Autodesk Inventor part; units mm, degrees
ref_plane "Plan de construction1" through (-33.0415, -128.424, -137.979) normal (0, -1, 0) x (1, 0, 0)
ref_plane "YZ Plane" through (0, 0, 0) normal (1, 0, 0) x (0, 1, 0)
ref_plane "XZ Plane" through (0, 0, 0) normal (0, 1, 0) x (-1, 0, 0)
sketch "Esquisse1" plane through (0, 0, 0) normal (0, 0, 1) x (1, 0, 0)
  circle A0 centre (-5.13, -4.2) radius 1.738
  circle A1 centre (43.13, -2.93) radius 1.738
  circle A2 centre (10.11, -55) radius 1.738
  circle A3 centre (51.1638, -91.424) radius 1.5682
  circle A4 centre (-13.5548, -91.424) radius 1.5682
  line L0 (-5.13, -4.2) -> (43.13, -2.93) construction
  line L1 (-5.0248, -8.1986) -> (43.2352, -6.9286)
  line L2 (43.0248, 1.0686) -> (-5.2352, -0.2014)
  arc A5 (-5.2352, -0.2014) -> (-5.0248, -8.1986) centre (-5.13, -4.2) ccw
  arc A6 (43.2352, -6.9286) -> (43.0248, 1.0686) centre (43.13, -2.93) ccw
  arc A7 (-1.2987, -3.0506) -> (-8.9613, -5.3494) centre (-5.13, -4.2) ccw
  arc A8 (46.508, -5.0722) -> (39.752, -0.7878) centre (43.13, -2.93) ccw
  arc A9 (-16.909, -89.2447) -> (-10.2005, -93.6032) centre (-13.5548, -91.424) ccw
  arc A10 (48.5091, -94.4161) -> (53.8185, -88.4319) centre (51.1638, -91.424) ccw
  line L3 (43.13, -2.93) -> (51.1638, -91.424) construction
  line L4 (39.1464, -3.2916) -> (47.1802, -91.7856)
  line L5 (55.1474, -91.0623) -> (47.1136, -2.5684)
  arc A11 (47.1136, -2.5684) -> (39.1464, -3.2916) centre (43.13, -2.93) ccw
  arc A12 (47.1802, -91.7856) -> (55.1474, -91.0623) centre (51.1638, -91.424) ccw
  line L6 (-5.13, -4.2) -> (-13.5548, -91.424) construction
  line L7 (-1.1485, -4.5846) -> (-9.5733, -91.8085)
  line L8 (-17.5362, -91.0394) -> (-9.1115, -3.8154)
  arc A13 (-1.1485, -4.5846) -> (-9.1115, -3.8154) centre (-5.13, -4.2) ccw
  arc A14 (-17.5362, -91.0394) -> (-9.5733, -91.8085) centre (-13.5548, -91.424) ccw
  line L9 (-13.5548, -91.424) -> (51.1638, -91.424) construction
  line L10 (-13.5548, -95.424) -> (51.1638, -95.424)
  line L11 (51.1638, -87.424) -> (-13.5548, -87.424)
  arc A15 (-13.5548, -87.424) -> (-13.5548, -95.424) centre (-13.5548, -91.424) ccw
  arc A16 (51.1638, -95.424) -> (51.1638, -87.424) centre (51.1638, -91.424) ccw
  point P0 (0, 0)
  point P1 (19, -3.565)
  point P2 (2.49, -29.6)
  point P3 (-1.7224, -73.212)
  point P4 (30.6369, -73.212)
  point P5 (47.1469, -47.177)
  point P6 (-9.3424, -47.812)
  point P7 (18.8045, -91.424)
  point P8 (39.4855, -7.0273)
  point P9 (46.7842, -87.424)
  point P10 (-9.1498, -87.424)
  point P11 (-1.4886, -8.1056)
  point P12 (-9.1115, -3.8154)
  point P13 (51.1638, -95.424)
  point P14 (47.1136, -2.5684)
  dimension "d2" = 8
  dimension "d3" = 8
  dimension "d5" = 8
  dimension "d6" = 8
extrude "Extrusion1" add sketch "Esquisse1" along normal blind 4 contours A5 A7 A13 L7 L1 | L1 L7 L11 A15 A9 L8 A5 | L7 A13 A7 L2 A8 A11 L4 L1 | L4 A11 A8 A6 L1 | L1 A6 L5 A10 A16 L11 L4 | L11 L4 A12 A10 L10 A9 A14 L7 | L7 A14 A9 A15 L11 | L11 A16 A10 A12 L4
fillet "Congé1" radius 19 2 edges at (-1.4886, -8.1056, 2) (39.4855, -7.0273, 2)
sketch "Esquisse2" plane through (0, 0, 0) normal (0, 0, -1) x (-1, 0, 0)
  arc A0 (9.1115, -3.8154) -> (5.2352, -0.2014) centre (5.13, -4.2) ccw
  line L0 (-43.0248, 1.0686) -> (5.2352, -0.2014)
  arc A1 (-43.0248, 1.0686) -> (-47.1136, -2.5684) centre (-43.13, -2.93) ccw
  line L1 (-55.1474, -91.0623) -> (-47.1136, -2.5684)
  arc A2 (-55.1474, -91.0623) -> (-51.1638, -95.424) centre (-51.1638, -91.424) ccw
  line L2 (13.5548, -95.424) -> (-51.1638, -95.424)
  arc A3 (13.5548, -95.424) -> (17.5362, -91.0394) centre (13.5548, -91.424) ccw
  line L3 (9.1115, -3.8154) -> (17.5362, -91.0394)
  arc A4 (-21.6744, -7.496) -> (-41.0964, -24.7716) centre (-22.1742, -26.4894) ccw
  line L4 (-15.3081, -7.6635) -> (-21.6744, -7.496)
  arc A5 (3.104, -24.8303) -> (-15.3081, -7.6635) centre (-15.808, -26.657) ccw
  line L5 (9.1498, -87.424) -> (3.104, -24.8303)
  line L6 (-46.7842, -87.424) -> (9.1498, -87.424)
  line L7 (-41.0964, -24.7716) -> (-46.7842, -87.424)
  circle A6 centre (5.13, -4.2) radius 1.738
  circle A7 centre (13.5548, -91.424) radius 1.5682
  circle A8 centre (-43.13, -2.93) radius 1.738
  circle A9 centre (-51.1638, -91.424) radius 1.5682
  line L8 (-41.0964, -24.7716) -> (-46.7842, -87.424)
  line L9 (-46.7842, -87.424) -> (-47.5105, -95.424)
  line L10 (-55.1474, -91.0623) -> (-47.1136, -2.5684)
  line L11 (-46.7842, -87.424) -> (9.1498, -87.424)
  line L12 (-46.7842, -87.424) -> (-54.8171, -87.424)
  line L13 (9.1498, -87.424) -> (9.9225, -95.424)
  line L14 (9.1498, -87.424) -> (17.187, -87.424)
  point P0 (0, 0)
extrude "Extrusion2" add sketch "Esquisse2" along normal blind 20 contours L3 A3 L2 L13 L14 | L9 L2 A2 L1 L12
sketch "Esquisse3" plane through (-13.5548, -95.424, 4) normal (0, -1, 0) x (1, 0, 0)
  line L0 (3.6323, -4) -> (61.0652, -4)
  line L1 (61.0652, -4) -> (61.0652, -24)
  line L2 (64.7185, -24) -> (61.0652, -24)
  line L3 (64.7185, -24) -> (64.7185, 0)
  line L4 (0, 0) -> (64.7185, 0)
  line L5 (0, -24) -> (0, 0)
  line L6 (3.6323, -24) -> (0, -24)
  line L7 (3.6323, -4) -> (3.6323, -24)
  line L8 (0, -24) -> (0, 0)
  line L9 (-3.9815, 0) -> (0, 0)
  line L10 (-3.9815, -24) -> (-3.9815, 0)
  line L11 (0, -24) -> (-3.9815, -24)
  line L12 (68.7022, -24) -> (68.7022, 0)
  line L13 (64.7185, 0) -> (68.7022, 0)
  line L14 (64.7185, -24) -> (64.7185, 0)
  line L15 (68.7022, -24) -> (64.7185, -24)
  point P0 (13.5548, -4)
  point P1 (0, 0)
  point P2 (64.7185, 0)
extrude "Extrusion3" add sketch "Esquisse3" along normal blind 25
sketch "Esquisse4" plane through (0, 0, 4) normal (0, 0, 1) x (1, 0, 0)
  arc A0 (-5.2352, -0.2014) -> (-9.1115, -3.8154) centre (-5.13, -4.2) ccw
  line L0 (-9.1115, -3.8154) -> (-17.5362, -91.0394)
  arc A1 (-17.5362, -91.0394) -> (-13.5548, -95.424) centre (-13.5548, -91.424) ccw
  line L1 (-13.5548, -95.424) -> (-17.5362, -95.424)
  line L2 (-17.5362, -95.424) -> (-17.5362, -120.424)
  line L3 (55.1474, -120.424) -> (-17.5362, -120.424)
  line L4 (55.1474, -95.424) -> (55.1474, -120.424)
  line L5 (55.1474, -95.424) -> (51.1638, -95.424)
  arc A2 (51.1638, -95.424) -> (55.1474, -91.0623) centre (51.1638, -91.424) ccw
  line L6 (55.1474, -91.0623) -> (47.1136, -2.5684)
  arc A3 (47.1136, -2.5684) -> (43.0248, 1.0686) centre (43.13, -2.93) ccw
  line L7 (43.0248, 1.0686) -> (-5.2352, -0.2014)
  line L8 (41.0964, -24.7716) -> (46.7842, -87.424)
  line L9 (46.7842, -87.424) -> (-9.1498, -87.424)
  line L10 (-9.1498, -87.424) -> (-3.104, -24.8303)
  arc A4 (15.3081, -7.6635) -> (-3.104, -24.8303) centre (15.808, -26.657) ccw
  line L11 (15.3081, -7.6635) -> (21.6744, -7.496)
  arc A5 (41.0964, -24.7716) -> (21.6744, -7.496) centre (22.1742, -26.4894) ccw
  circle A6 centre (-5.13, -4.2) radius 1.738
  circle A7 centre (-13.5548, -91.424) radius 1.5682
  circle A8 centre (43.13, -2.93) radius 1.738
  circle A9 centre (51.1638, -91.424) radius 1.5682
  line L12 (-17.5362, -91.0394) -> (-17.187, -87.424)
  line L13 (-17.5362, -95.424) -> (-17.5362, -91.0394)
  line L14 (55.1474, -91.0623) -> (55.1474, -95.424)
  point P0 (0, 0)
  point P1 (55.1474, -91.7856)
  point P2 (-17.5362, -91.8085)
extrude "Extrusion4" add sketch "Esquisse4" against normal up to surface (24 mm away) contours A1 L1 L13 | L14 L5 A2
sketch "Esquisse5" plane through (-13.5548, -120.424, 4) normal (0, -1, 0) x (1, 0, 0)
  line L0 (68.7022, 0) -> (-3.9815, 0)
  line L1 (-3.9815, 0) -> (-3.9815, -24)
  line L2 (68.7022, 0) -> (-3.9815, 0)
  line L3 (-3.9815, 0) -> (-3.9815, -24)
  line L4 (-3.9815, -24) -> (68.7022, -24)
  line L5 (68.7022, -24) -> (68.7022, 0)
  point P0 (13.5548, -4)
extrude "Extrusion5" add sketch "Esquisse5" along normal blind 3
sketch "Esquisse6" plane through (-13.5548, -120.424, 4) normal (0, 1, 0) x (1, 0, 0)
  circle A0 centre (52.3133, 6.979) radius 1.6
  circle A1 centre (52.3133, 16.979) radius 1.6
  circle A2 centre (42.3133, 16.979) radius 1.6
  circle A3 centre (42.3133, 6.979) radius 1.6
  circle A4 centre (32.3133, 6.979) radius 1.6
  circle A5 centre (32.3133, 16.979) radius 1.6
  circle A6 centre (22.3133, 16.979) radius 1.6
  circle A7 centre (22.3133, 6.979) radius 1.6
  circle A8 centre (12.3133, 6.979) radius 1.6
  circle A9 centre (12.3133, 16.979) radius 1.6
  point P0 (13.5548, 4)
ref_plane "Plan de construction1" through (-33.0415, -128.424, -137.979) normal (0, -1, 0) x (1, 0, 0)
extrude "Extrusion6" cut sketch "Esquisse6" against normal up to surface (8 mm away)
properties part number "holder"
Verification items for the finished model (mm, model axes). A direction names the side the tool comes from. Give positions to 0.01 mm unless a question says otherwise; leave off trailing zeros. Write each loop counter-clockwise with the first axis right and the second up, starting at its lowest first coordinate (ties: lowest second). Pieces come first, ordered by that corner, then holes. Notation, with made-up numbers: M 31.25,79.5 L 79.25,79.5 A22 cw 79.25,86.5 Z; hole C 87,-23.5 d10. An arc over 180 degrees is marked long. Write item = value, one per line.
(1) Sectioned sample at A-A (y = -115). Record the cut outline in (x, z).
Found:
outline = M -17.54,-20 L -9.92,-20 L -9.92,0 L 47.51,0 L 47.51,-20 L 55.15,-20 L 55.15,4 L -17.54,4 Z
(2) Go/stop test with flat-tipped pins: pin 1 Ø6 at (y, z) = (-113.5, -7.5) entering from +X; pin 2 Ø4 at (x, z) = (38.76, -2.98) entering from -Y; pin 3 Ø4 at (x, z) = (-12, -15) entering from +Y; pin 4 Ø4.5 at (x, y) = (-5.13, -4.2) entering from -Z. Record where each tip stops, or that it passes through.
Found:
pin_1 = 55.15
pin_2 = -123.42
pin_3 = -87.42
pin_4 = 0
(3) Sectioned sample at D-D (y = -85). Record the cut outline in (x, z).
Found:
outline = M -16.95,0 L -8.92,0 L -8.92,4 L -16.95,4 Z; M 46.56,0 L 54.6,0 L 54.6,4 L 46.56,4 Z
(4) Access from +Z, -Z, +X, -X, +Y, -Y to the whole of each face (thin tool, end or side, straight path). Record for faces 4 (the face through (30, -87.424, 1)), 5 (the face through (-13, -87.424, -10)), 6 (the face through (34.951, -12.427, 2.028)).
Found:
face_4 = -Z
face_5 = -Z, +X, -X, +Y
face_6 = +Z, -Z
(5) Sectioned sample at C-C (z = -18.5). Give the number of separate pieces and of enclosed holes in the cut face, then the cut area to 3 significant figures.
Found:
separate_pieces = 1
enclosed_holes = 2
area = 711 mm2
(6) Draft check along Z on faces 1 (the face through (18, -104, 0)), 2 (the face through (-1.588, -121.903, -11.417)), 3 (the face through (-6.085, -55.689, 1.972)). Enter one of: released by +Z, released by -Z, zero draft, split by the parting line, or undercut.
Found:
face_1 = released by -Z
face_2 = undercut
face_3 = zero draft
(7) Material ranges on line 1 (X direction, y = -91, z = 2) (3 decimals); line 2 (Z direction, x = 44, y = -47.5); line 3 (X direction, y = -116, z = -2.25), recorded low to high.
Found:
line_1 = -17.532 to -15.065, -12.045 to 49.654, 52.674 to 55.142
line_2 = 0 to 4
line_3 = -17.54 to -9.92, 47.51 to 55.15
(8) Sectioned sample at B-B (y = -21.5). Record the cut outline in (x, z), then the cut area to 3 significant figures.
Found:
outline = M -10.82,0 L -2.48,0 L -2.48,4 L -10.82,4 Z; M 40.51,0 L 48.83,0 L 48.83,4 L 40.51,4 Z
area = 66.7 mm2
